from build123d import *

# Parameters (mm, degrees)
BOSS_EXTRUDE1_DEPTH = 3


with BuildPart() as part:
    # Sketch1 → Boss-Extrude1 (new body)
    with BuildSketch(Plane.XY):
        with BuildLine():
            Line((0, 0), (10, 0))
            Line((10, 0), (10, 3))
            Line((10, 3), (30, 3))
            Line((30, 3), (30, 0))
            Line((30, 0), (100, 0))
            Line((100, 0), (100, 3))
            Line((100, 3), (120, 3))
            Line((120, 3), (120, 0))
            Line((120, 0), (130, 0))
            Line((130, 0), (130, -25))
            Line((130, -25), (117.75, -25))
            Line((117.75, -25), (117.75, -10))
            ThreePointArc((117.75, -10), (113.75, -6), (109.75, -10))
            Line((109.75, -10), (109.75, -25))
            Line((109.75, -25), (69.19, -25))
            Line((69.19, -25), (69.19, -12))
            ThreePointArc((69.19, -12), (65.09, -7.9), (60.99, -12))
            Line((60.99, -12), (60.99, -25))
            Line((60.99, -25), (20.25, -25))
            Line((20.25, -25), (20.25, -10))
            ThreePointArc((20.25, -10), (16.25, -6), (12.25, -10))
            Line((12.25, -10), (12.25, -25))
            Line((12.25, -25), (0, -25))
            Line((0, -25), (0, 0))
        make_face()
    extrude(amount=BOSS_EXTRUDE1_DEPTH)


solid = part.part
Verification items for the finished model (mm, model axes). A direction names the side the tool comes from. Give positions to 0.01 mm unless a question says otherwise; leave off trailing zeros. Write each loop counter-clockwise with the first axis right and the second up, starting at its lowest first coordinate (ties: lowest second). Pieces come first, ordered by that corner, then holes. Notation, with made-up numbers: M 52.25,41.25 L 108.25,41.25 A18 cw 108.25,66.25 Z; hole C 3.25,46 d9. An arc over 180 degrees is marked long. Put each result on its own line as item: value. Start each with the question number.
1. Section check C-C (x = 92.5). Record the cut outline in (y, z), and give its area (3 significant figures).
2. Section check A-A (z = 0.5). Record the cut outline in (x, y).
3. Section check B-B (x = 16.25). Record the cut outline in (y, z), and give its area (3 significant figures).
4. Set-up check for faces 5 (the face through (120, 2, 1)), 6 (the face through (30, 2, 1)), 7 (the face through (117.75, -18, 1)), 8 (the face through (10, 1, 1)): record each of +Z, -Z, +X, -X, +Y, -Y from which the full face is reachable in a straight line by a thin tool's end or side.
5. Scan lines: line 1 along X through (y, z) = (-16, 1.4); line 2 along X through (y, z) = (0.25, 2.7); line 3 along Y through (x, z) = (9, 1.3). Record each from-to range of solid material in increasing order. Write a range as [from, to].
6. Go/stop test with flat-tipped pins: pin 1 Ø1.5 at (y, z) = (-20, 1.5) entering from -X; pin 2 Ø0.9 at (y, z) = (1.5, 1.5) entering from +X; pin 3 Ø0.9 at (x, z) = (122.5, 1.5) entering from +Y. Record where each tip stops, or that it passes through.
7. Draft check along X on faces 1 (the face through (109.75, -17, 1)), 2 (the face through (65.9, -7.7, 3)), 3 (the face through (0, -13, 1)), 4 (the face through (12.25, -17, 1)). Enter one of: +X half, -X half, draft (parallel to the pull), parting line (faces both ways), or undercut.
Answer list:
1. outline: M -25,0 L 0,0 L 0,3 L -25,3 Z
1. area: 75.0 mm2
2. outline: M 0,-25 L 12.25,-25 L 12.25,-10 A4 cw 20.25,-10 L 20.25,-25 L 60.99,-25 L 60.99,-12 A4.1 cw 69.19,-12 L 69.19,-25 L 109.75,-25 L 109.75,-10 A4 cw 117.75,-10 L 117.75,-25 L 130,-25 L 130,0 L 120,0 L 120,3 L 100,3 L 100,0 L 30,0 L 30,3 L 10,3 L 10,0 L 0,0 Z
3. outline: M -6,0 L 3,0 L 3,3 L -6,3 Z
3. area: 27.0 mm2
4. face 5: +Z, -Z, +X, +Y
4. face 6: +Z, -Z, +Y
4. face 7: +Z, -Z, -Y
4. face 8: +Z, -Z, -X, +Y
5. line 1: [0, 12.25], [20.25, 60.99], [69.19, 109.75], [117.75, 130]
5. line 2: [10, 30], [100, 120]
5. line 3: [-25, 0]
6. pin 1: x = 0
6. pin 2: x = 120
6. pin 3: y = 0
7. face 1: undercut
7. face 2: draft
7. face 3: -X half
7. face 4: undercut
